Print and shaded views of the part. All mm, measured from the part's lowest x, y and z. A direction names the side the tool comes from. Give positions to 0.01 mm unless a question says otherwise; leave off trailing zeros. Loops run counter-clockwise (first coordinate to the right, second up) from the corner with the lowest first, then second, coordinate; pieces in that order, holes last. Notation, with made-up numbers: M 14.25,-2.75 L 62.25,-2.75 A26 cw 62.25,15.25 Z; hole C 13.25,21.5 d10. An arc over 180 degrees is marked long. Answer as CSV lines item,"result".
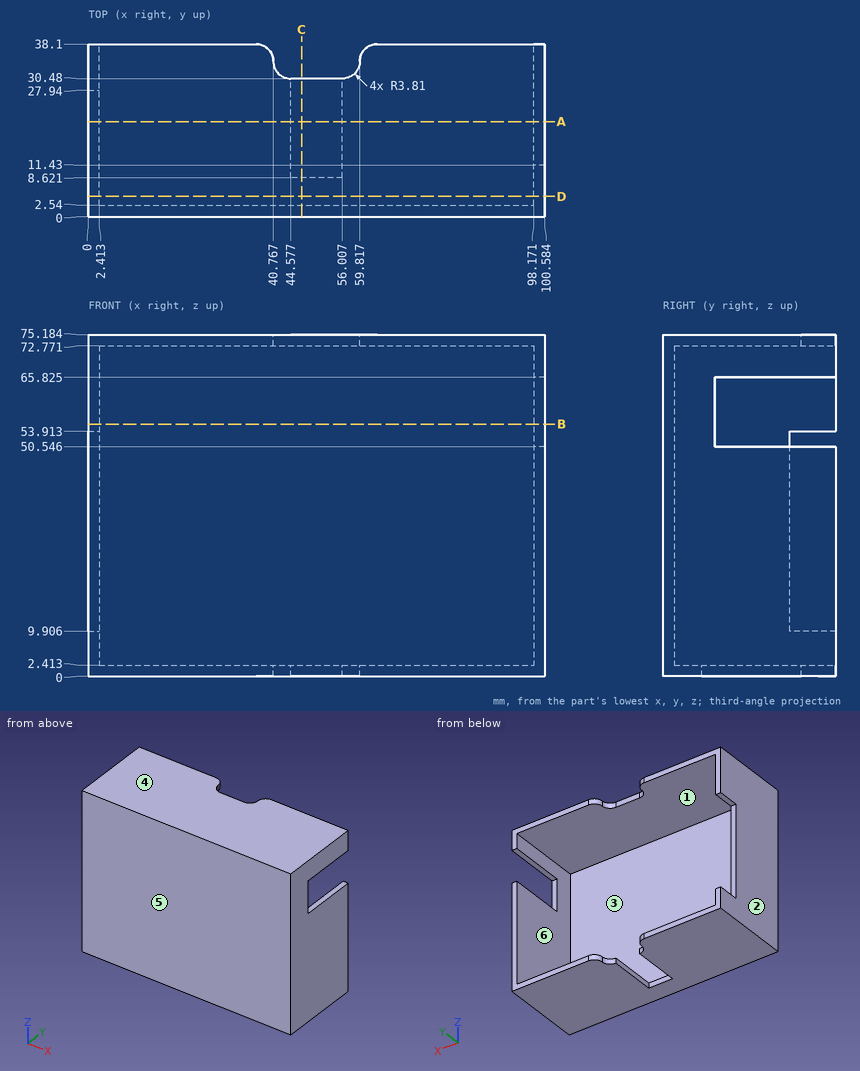
Q1. Cut at D-D (y = 4.5). Write the cut outline in (x, z), and give its area (3 significant figures).
Solution:
outline,"M 0,0 L 100.58,0 L 100.58,75.18 L 0,75.18 Z; hole M 2.41,2.41 L 98.17,2.41 L 98.17,72.77 L 2.41,72.77 Z"
area,"825 mm²"
Q2. Cut at B-B (z = 55.5). Write the cut outline in (x, y), and give its area (3 significant figures).
Solution:
outline,"M 0,0 L 100.58,0 L 100.58,11.43 L 98.17,11.43 L 98.17,2.54 L 2.41,2.54 L 2.41,38.1 L 0,38.1 Z"
area,"363 mm²"
Q3. Which spindle directions (+Z, -Z, +X, -X, +Y, -Y) get a long thin tool onto all of the face, cutting with end or side? Do the marked faces 5 and 6. Say none if no direction does.
Solution:
face 5,"+Z, -Z, +X, -X, -Y"
face 6,"+Y"
Q4. Cut at C-C (x = 47). Write the cut outline in (y, z).
Solution:
outline,"M 0,0 L 8.62,0 L 8.62,2.41 L 2.54,2.41 L 2.54,72.77 L 30.48,72.77 L 30.48,75.18 L 0,75.18 Z"
Q5. Mould opens along X. For the marked faces 1, 2, 3 and 4 say: released by +X, released by -X, zero draft, split by the parting line, or undercut.
Solution:
face 1,"undercut"
face 2,"released by -X"
face 3,"undercut"
face 4,"zero draft"
Q6. Pin check, flat tips, straight feed: P1, Ø1.9, axis at x = 49.5, z = 1, coming from the +Y side; P2, Ø1, axis at x = 51, y = 19.5, coming from the -Z side; P3, Ø1, axis at x = 35.5, z = 62.5, coming from the +Y side. Stop position of each tip, or through.
Solution:
P1,"stops at y = 8.62"
P2,"stops at z = 72.77"
P3,"stops at y = 2.54"
Q7. Cut at A-A (y = 21). Write the cut outline in (x, z) (1 decimal).
Solution:
outline,"M 0,0 L 44.6,0 L 44.6,2.4 L 2.4,2.4 L 2.4,72.8 L 98.2,72.8 L 98.2,65.8 L 100.6,65.8 L 100.6,75.2 L 0,75.2 Z; M 56,0 L 100.6,0 L 100.6,50.5 L 98.2,50.5 L 98.2,2.4 L 56,2.4 Z"
Q8. Wall check: line 1 (X direction, y = 21, z = 20); line 2 (Z direction, x = 40.5, y = 6); line 3 (Y direction, x = 76, z = 22). Give the ranges that are in metal, low to high. Write a range as [from, to].
Solution:
line 1,"x = [0, 2.41], [98.17, 100.58]"
line 2,"z = [0, 2.41], [72.77, 75.18]"
line 3,"y = [0, 2.54]"
